Geometry check sheet. Reference: the model listing, model coordinates, mm. A direction names the side the tool comes from. Give positions to 0.01 mm unless a question says otherwise; leave off trailing zeros. Loops run counter-clockwise (first coordinate to the right, second up) from the corner with the lowest first, then second, coordinate; pieces in that order, holes last. Notation, with made-up numbers: (-29.5, -26.5) -> (0.5, -26.5) arc R16 cw to (0.5, -19.5) -> close; hole circle Ø1 at (30, 66.5). An arc over 180 degrees is marked (long way). Write item = value, one per line.
```python
from build123d import *

# Parameters (mm, degrees)
SKETCH1_R               = 8
SKETCH1_R_2             = 4
BOSS_EXTRUDE1_DEPTH     = 30
SKETCH2_R               = 4.5
SKETCH2_R_2             = 1.5
BOSS_EXTRUDE2_DEPTH     = 4
FILLET1_R               = 7
SKETCH3_R               = 5
SKETCH3_R_2             = 1.5
BOSS_EXTRUDE3_DEPTH     = 4
FILLET2_R               = 7
SKETCH4_R               = 3.25
CUT_EXTRUDE1_DEPTH      = 10
CHAMFER1_SIZE           = 1
CUT_EXTRUDE2_DEPTH      = 1.5
CUT_EXTRUDE2_DEPTH_BACK = 1.5
CHAMFER2_SIZE           = 1.732050808
CHAMFER2_SIZE_2         = 1
CHAMFER3_SIZE           = 1.732050808
CHAMFER3_SIZE_2         = 1


with BuildPart() as part:
    # Sketch1 → Boss-Extrude1 (new body)
    with BuildSketch(Plane(origin=(0, 0, 0), x_dir=(1, 0, 0), z_dir=(0, 1, 0))):
        with Locations(Location((0, 0, 0), (0, 0, 270))):
            Circle(SKETCH1_R)
        with Locations(Location((0, 0, 0), (0, 0, 270))):
            Circle(SKETCH1_R_2, mode=Mode.SUBTRACT)
    extrude(amount=BOSS_EXTRUDE1_DEPTH)

    # Sketch2 → Boss-Extrude2 (add)
    # profile 1 of 2: a face of its own
    with BuildSketch(Plane(origin=(0, 30, 0), x_dir=(1, 0, 0), z_dir=(0, 1, 0))):
        with Locations((-10, 0)):
            Circle(SKETCH2_R)
        with Locations(Location((-10, 0, 0), (0, 0, 270))):
            Circle(SKETCH2_R_2, mode=Mode.SUBTRACT)
    # profile 2 of 2: a face of its own
    with BuildSketch(Plane(origin=(0, 30, 0), x_dir=(1, 0, 0), z_dir=(0, 1, 0))):
        with Locations((10, 0)):
            Circle(SKETCH2_R)
        with Locations(Location((10, 0, 0), (0, 0, 90))):
            Circle(SKETCH2_R_2, mode=Mode.SUBTRACT)
    extrude(amount=-BOSS_EXTRUDE2_DEPTH)

    # Fillet1
    fillet1_edges = [part.edges().sort_by_distance(p)[0] for p in [
        (-7.1875, 28, 3.512811374),
        (-7.1875, 28, -3.512811374),
        (7.1875, 28, -3.512811374),
        (7.1875, 28, 3.512811374),
    ]]
    fillet(fillet1_edges, radius=FILLET1_R)

    # Sketch3 → Boss-Extrude3 (add)
    # profile 1 of 3: a face of its own
    with BuildSketch(Plane.XZ):
        with Locations((0, 10)):
            Circle(SKETCH3_R)
        with Locations(Location((0, 10, 0), (0, 0, 270))):
            Circle(SKETCH3_R_2, mode=Mode.SUBTRACT)
    # profile 2 of 3: a face of its own
    with BuildSketch(Plane.XZ):
        with Locations((8.660254038, -5)):
            Circle(SKETCH3_R)
        with Locations(Location((8.660254038, -5, 0), (0, 0, 270))):
            Circle(SKETCH3_R_2, mode=Mode.SUBTRACT)
    # profile 3 of 3: a face of its own
    with BuildSketch(Plane.XZ):
        with Locations((-8.660254038, -5)):
            Circle(SKETCH3_R)
        with Locations(Location((-8.660254038, -5, 0), (0, 0, 270))):
            Circle(SKETCH3_R_2, mode=Mode.SUBTRACT)
    extrude(amount=-BOSS_EXTRUDE3_DEPTH)

    # Fillet2
    fillet2_edges = [part.edges().sort_by_distance(p)[0] for p in [
        (3.962007067, 2, 6.95),
        (-3.962007067, 2, 6.95),
        (4.037873023, 2, -6.90619877),
        (7.99988009, 2, -0.04380123),
        (-7.99988009, 2, -0.04380123),
        (-4.037873023, 2, -6.90619877),
    ]]
    fillet(fillet2_edges, radius=FILLET2_R)

    # Sketch4 → Cut-Extrude1 (cut)
    with BuildSketch(Plane(origin=(0, 4, 0), x_dir=(1, 0, 0), z_dir=(0, 1, 0))):
        with Locations((8.660254038, 5)):
            Circle(SKETCH4_R)
        with Locations((0, -10)):
            Circle(SKETCH4_R)
        with Locations((-8.660254038, 5)):
            Circle(SKETCH4_R)
    extrude(amount=CUT_EXTRUDE1_DEPTH, mode=Mode.SUBTRACT)

    # Chamfer1
    chamfer1_edges = [part.edges().sort_by_distance(p)[0] for p in [
        (-6.92820323, 14, -4),
        (1.145643924, 14, 7.917543811),
        (6.92820323, 14, -4),
    ]]
    chamfer(chamfer1_edges, length=CHAMFER1_SIZE)

    # Sketch5 → Cut-Extrude2 (cut, two sides: drawn at the far end of the back side and taken through both)
    with BuildSketch(Plane.XZ.offset(-26).offset(-CUT_EXTRUDE2_DEPTH_BACK)):
        Polygon((-10, 3.175426481), (-12.75, 1.58771324), (-12.75, -1.58771324), (-10, -3.175426481), (-7.25, -1.58771324), (-7.25, 1.58771324), align=None)
        Polygon((7.25, 1.58771324), (10, 3.175426481), (12.75, 1.58771324), (12.75, -1.58771324), (10, -3.175426481), (7.25, -1.58771324), align=None)
    extrude(amount=CUT_EXTRUDE2_DEPTH + CUT_EXTRUDE2_DEPTH_BACK, mode=Mode.SUBTRACT)

    # Chamfer2
    # the kernel refuses this chamfer: 1.732050808, 1 mm, written as the material it takes off along each edge
    with BuildSketch(Plane(origin=(0, 24.5, 0), x_dir=(-0.6976791075699221, 0, 0.7164104011392053), z_dir=(0.7164104011392053, 0, 0.6976791075699221))) as chamfer2_piece_1_section:
        Polygon((8, CHAMFER2_SIZE), (8 - CHAMFER2_SIZE_2, 0), (8, 0), align=None)
    chamfer2_piece_1 = revolve(axis=Axis((0, 24.5, 0), (0, -1, 0)), revolution_arc=91.517812411, mode=Mode.PRIVATE)
    chamfer2_piece_1 = split(chamfer2_piece_1, bisect_by=Plane(origin=(-6.887741649, 23.854160996, 1.378563284), z_dir=(-0.5000000000000001, 0, -0.8660254037844386)), keep=Keep.TOP, mode=Mode.PRIVATE)
    chamfer2_piece_1 = split(chamfer2_piece_1, bisect_by=Plane(origin=(-7.25, 23.854160996, 0), z_dir=(-1, 0, 0)), keep=Keep.TOP, mode=Mode.PRIVATE)
    chamfer2_piece_1 = split(chamfer2_piece_1, bisect_by=Plane(origin=(-6.887741649, 23.854160996, -1.378563284), z_dir=(-0.49999999999999994, 0, 0.8660254037844389)), keep=Keep.TOP, mode=Mode.PRIVATE)
    add(chamfer2_piece_1, mode=Mode.SUBTRACT)

    # Chamfer3
    # the kernel refuses this chamfer: 1.732050808, 1 mm, written as the material it takes off along each edge
    with BuildSketch(Plane(origin=(0, 24.5, 0), x_dir=(0.6976791075699224, 0, -0.7164104011392051), z_dir=(-0.7164104011392051, 0, -0.6976791075699224))) as chamfer3_piece_1_section:
        Polygon((8, CHAMFER3_SIZE), (8 - CHAMFER3_SIZE_2, 0), (8, 0), align=None)
    chamfer3_piece_1 = revolve(axis=Axis((0, 24.5, 0), (0, -1, 0)), revolution_arc=91.517812411, mode=Mode.PRIVATE)
    chamfer3_piece_1 = split(chamfer3_piece_1, bisect_by=Plane(origin=(6.887741649, 23.854160996, -1.378563284), z_dir=(0.49999999999999994, 0, 0.8660254037844389)), keep=Keep.TOP, mode=Mode.PRIVATE)
    chamfer3_piece_1 = split(chamfer3_piece_1, bisect_by=Plane(origin=(7.25, 23.854160996, 0), z_dir=(1, 0, 0)), keep=Keep.TOP, mode=Mode.PRIVATE)
    chamfer3_piece_1 = split(chamfer3_piece_1, bisect_by=Plane(origin=(6.887741649, 23.854160996, 1.378563284), z_dir=(0.5000000000000001, 0, -0.8660254037844386)), keep=Keep.TOP, mode=Mode.PRIVATE)
    add(chamfer3_piece_1, mode=Mode.SUBTRACT)


solid = part.part
```
Item 1: Gauge pin test, flat ends, axial feed: pin 1 (4 mm diameter, centred on x = 6, z = 11, fed in from +Y); pin 2 (5 mm diameter, centred on x = -6, y = 22.5, fed in from -Z); pin 3 (12 mm diameter, centred on x = -6.5, y = 22, fed in from +Z). Record the tip position at first contact, or that the pin passes through.
Answer:
pin_1 = 4
pin_2 = -7.19
pin_3 = 7.98
Item 2: Tool access check on faces 1 (the flat face through (11.394, 26.76, -2.37)), 2 (the cylindrical face through (-5.863, 9.423, -3.345)), 3 (the cylindrical face through (5.828, 9.423, -3.406)), 4 (the flat face through (-12.75, 27, 0)). Record the directions out of +Z, -Z, +X, -X, +Y, -Y that give a thin tool (end or side, any length) a straight path to the whole face; none if there is none.
Answer:
face_1 = none
face_2 = -X
face_3 = +X
face_4 = -Y
Item 3: Section check A-A, the plane x = 0. Record the cut outline in (y, z).
Answer:
outline = (0, -8) -> (30, -8) -> (30, -4) -> (0, -4) -> close; (0, 4) -> (30, 4) -> (30, 8) -> (15, 8) -> (14, 7) -> (14, 6.75) -> (4, 6.75) -> (4, 8.5) -> (0, 8.5) -> close; (0, 11.5) -> (4, 11.5) -> (4, 15) -> (0, 15) -> close
Item 4: Section check B-B, the plane z = 10. Record the cut outline in (x, y).
Answer:
outline = (-5, 0) -> (-1.5, 0) -> (-1.5, 4) -> (-5, 4) -> close; (1.5, 0) -> (5, 0) -> (5, 4) -> (1.5, 4) -> close
Item 5: Section check C-C, the plane y = 25. Record the cut outline in (x, z), plus the area to 3 significant figures.
Answer:
outline = (-7.77, -1.89) arc R8 ccw to (7.77, -1.89) -> (7.25, -1.59) -> (7.25, 1.59) -> (7.77, 1.89) arc R8 ccw to (-7.77, 1.89) -> (-7.25, 1.59) -> (-7.25, -1.59) -> close; hole circle Ø8 at (0, 0)
area = 146 mm^2
Item 6: Section check D-D, the plane x = 12. Record the cut outline in (y, z), plus the area to 3 significant figures.
Answer:
outline = (0, -8.72) -> (4, -8.72) -> (4, -1.28) -> (0, -1.28) -> close; (26, -4.03) -> (30, -4.03) -> (30, 4.03) -> (26, 4.03) -> (26, 2.02) -> (27.5, 2.02) -> (27.5, -2.02) -> (26, -2.02) -> close
area = 56.0 mm^2
Item 7: Thickness scan on L1, parallel to X at y = 2.8, z = -5; L2, parallel to X at y = 29.4, z = 0; L3, parallel to Z at x = 0.25, y = 6.5. Record the ranges inside material, lowest first. Write a range as [from, to].
Answer:
L1 = [-13.66, -10.16], [-7.16, 7.16], [10.16, 13.66]
L2 = [-14.5, -11.5], [-8.5, -4], [4, 8.5], [11.5, 14.5]
L3 = [-8, -3.99], [3.99, 6.76]
Item 8: Draft check along Z on faces 5 (the cylindrical face through (12.93, 1.97, -7.6)), 6 (the conical face through (0, 14.5, 7.5)), 7 (the flat face through (-11.3, 27.5, -1.4)). Enter one of: +Z half, -Z half, draft (parallel to the pull), parting line (faces both ways), or undercut.
Answer:
face_5 = parting line
face_6 = +Z half
face_7 = undercut
